from build123d import *

# Parameters (mm, degrees)
SKETCH1_W           = 1016
SKETCH1_H           = 406.4
BOSS_EXTRUDE1_DEPTH = 6.35
BOSS_EXTRUDE2_DEPTH = 1016


with BuildPart() as part:
    # Sketch1 → Boss-Extrude1 (new body)
    with BuildSketch(Plane(origin=(0, 0, 0), x_dir=(1, 0, 0), z_dir=(0, 1, 0))):
        with Locations((508, 203.2)):
            Rectangle(SKETCH1_W, SKETCH1_H)
    extrude(amount=BOSS_EXTRUDE1_DEPTH)

    # Sketch2 → Boss-Extrude2 (add)
    with BuildSketch(Plane(origin=(0, 0, 0), x_dir=(0, 0, -1), z_dir=(1, 0, 0))):
        Polygon((0, 0), (-36.378303543, 35.457848656), (-33.204345912, 38.714199465), (0, 6.35), align=None)
        Polygon((406.4, 6.35), (406.4, 0), (442.778303543, 35.457848656), (439.604345912, 38.714199465), align=None)
    extrude(amount=BOSS_EXTRUDE2_DEPTH)


solid = part.part
Could you check a few things on this model? Use its own coordinates, in mm. A direction names the side the tool comes from. Give positions to 0.01 mm unless a question says otherwise; leave off trailing zeros. Order: outer loops, then holes, each group sorted by start corner. A loop starts at its lowest first (then second) coordinate and runs counter-clockwise, first axis right, second up. Notation, with made-up numbers: (16, 56) -> (23, 56) arc R13 cw to (23, 75) -> close; hole circle Ø8 at (-35, -18). An arc over 180 degrees is marked (long way). Answer in a Markdown table with one row per item. Add a question column.
Item 1: We'd pull the mould along Z, two halves only. Please class faces 3 (the flat face through (500.888, 17.481, 17.935)), 4 (the flat face through (1016, 5, -204)), 5 (the flat face through (501, 6.35, -206)), 6 (the flat face through (500.888, 22.759, -423.235)): pulls with the +Z half, pulls with the -Z half, needs draft (parallel to the pull), parting line crosses it, or undercut.
Item 2: For faces 1 (the flat face through (500.888, 22.759, 16.835)), 2 (the flat face through (501, 0, -206)), which set-ups out of +Z, -Z, +X, -X, +Y, -Y let a thin tool reach every point of the face, with its end or its side?
Item 3: Imagine slicing it at A-A (y = 16). List the corners of the cut face in (x, z) for me.
Item 4: Imagine slicing it at B-B (x = 274). List the corners of the cut face in (y, z) for me.
Item 5: I'm going to push flat-ended pins straight in: P1, Ø10, axis at x = 466.5, z = -59.5, coming from the +Y side; P2, Ø3, axis at x = 792.5, z = -12, coming from the -Y side. Where does each tip first touch, or does it pass through?
Item 6: Please list where these lines run through material, in increasing order: probe 1 along Y at (x, z) = (564.5, -358.5); probe 2 along Z at (x, y) = (800, 8); probe 3 along Z at (x, y) = (110.5, 26).
Item 7: Imagine slicing it at C-C (z = -109). List the corners of the cut face in (x, y) for me, and give its area (3 significant figures).
Result:
| question | item | result |
|---|---|---|
| 1 | face 3 | pulls with the +Z half |
| 1 | face 4 | needs draft |
| 1 | face 5 | undercut |
| 1 | face 6 | undercut |
| 2 | face 1 | +X, -X, +Y |
| 2 | face 2 | +Z, -Z, +X, -X, -Y |
| 3 | outline | (0, -422.82) -> (1016, -422.82) -> (1016, -416.3) -> (0, -416.3) -> close; (0, 9.9) -> (1016, 9.9) -> (1016, 16.42) -> (0, 16.42) -> close |
| 4 | outline | (0, -406.4) -> (35.46, -442.78) -> (38.71, -439.6) -> (6.35, -406.4) -> (6.35, 0) -> (38.71, 33.2) -> (35.46, 36.38) -> (0, 0) -> close |
| 5 | P1 | y = 6.35 |
| 5 | P2 | y = 0 |
| 6 | probe 1 | 0 to 6.35 |
| 6 | probe 2 | -414.61 to -408.09, 1.69 to 8.21 |
| 6 | probe 3 | -433.07 to -426.56, 20.16 to 26.67 |
| 7 | outline | (0, 0) -> (1016, 0) -> (1016, 6.35) -> (0, 6.35) -> close |
| 7 | area | 6,450 mm2 |
